```python
from build123d import *

# Parameters (mm, degrees)
SKETCH_1_R          = 210
SKETCH_1_R_2        = 203
EXTRUDE_2_DEPTH     = 174
EXTRUDE_START       = -174
EXTRUDE_4_DEPTH     = 174
CUT_EXTRUDE_1_DEPTH = 654
EXTRUDE_5_DEPTH     = 174
EXTRUDE_6_DEPTH     = 174
EXTRUDE_7_DEPTH     = 174
EXTRUDE_8_DEPTH     = 174
EXTRUDE_9_DEPTH     = 174
SKETCH_11_R         = 55
CUT_EXTRUDE_4_DEPTH = 221.5
CUT_EXTRUDE_5_DEPTH = 87


with BuildPart() as part:
    # 草图1 → 凸台-拉伸2 (new body)
    with BuildSketch(Plane.XY):
        Circle(SKETCH_1_R)
        Circle(SKETCH_1_R_2, mode=Mode.SUBTRACT)
    extrude(amount=EXTRUDE_2_DEPTH)

    # 草图2 → 凸台-拉伸4 (add)
    with BuildSketch(Plane.XY.offset(174).offset(EXTRUDE_START)):
        with BuildLine():
            Line((-170.735431044, -102), (-173.735431044, -102))
            Line((-173.735431044, -102), (-175.513532242, -102))
            ThreePointArc((-175.513532242, -102), (-174.63092392, -103.50381834), (-173.735431044, -105))
            Line((-173.735431044, -105), (-170.735431044, -105))
            Line((-170.735431044, -105), (-170.735431044, -102))
        make_face()
        with BuildLine():
            ThreePointArc((173.735431044, -105), (174.63092392, -103.50381834), (175.513532242, -102))
            Line((175.513532242, -102), (173.735431044, -102))
            Line((173.735431044, -102), (170.735431044, -102))
            Line((170.735431044, -102), (170.735431044, -105))
            Line((170.735431044, -105), (173.735431044, -105))
        make_face()
    extrude(amount=EXTRUDE_4_DEPTH)

    # 草图3 → 切除-拉伸1 (cut)
    with BuildSketch(Plane.XY.offset(174)):
        Polygon((-170.735431044, -102), (238.333646515, -102), (254.334169784, 272.292523591), (-334.569415043, 221.85110305), (-306.830562533, -102), align=None)
    extrude(amount=-CUT_EXTRUDE_1_DEPTH, mode=Mode.SUBTRACT)

    # 草图5 → 凸台-拉伸5 (add)
    with BuildSketch(Plane.XY.offset(174).offset(EXTRUDE_START)):
        with BuildLine():
            Line((-120, -209.75), (-10.243900624, -209.75))
            ThreePointArc((-10.243900624, -209.75), (-67.755470707, -198.769203322), (-120, -172.336879396))
            Line((-120, -172.336879396), (-120, -209.75))
        make_face()
        with BuildLine():
            ThreePointArc((120, -172.336879396), (67.755470707, -198.769203322), (10.243900624, -209.75))
            Line((10.243900624, -209.75), (120, -209.75))
            Line((120, -209.75), (120, -172.336879396))
        make_face()
    extrude(amount=EXTRUDE_5_DEPTH)

    # 草图6 → 凸台-拉伸6 (add)
    with BuildSketch(Plane.XY.offset(174).offset(EXTRUDE_START)):
        with BuildLine():
            Line((-175.513532242, -102), (-166.195667814, -102))
            ThreePointArc((-166.195667814, -102), (0, -195), (166.195667814, -102))
            Line((166.195667814, -102), (175.513532242, -102))
            ThreePointArc((175.513532242, -102), (0, -203), (-175.513532242, -102))
        make_face()
    extrude(amount=EXTRUDE_6_DEPTH)

    # 草图7 → 凸台-拉伸7 (add)
    with BuildSketch(Plane.XY.offset(174).offset(EXTRUDE_START)):
        with BuildLine():
            Line((-166.933126535, -92), (-166.933126535, -95))
            Line((-166.933126535, -95), (-170.293863659, -95))
            ThreePointArc((-170.293863659, -95), (0, -195), (170.293863659, -95))
            Line((170.293863659, -95), (166.933126535, -95))
            Line((166.933126535, -95), (166.933126535, -92))
            Line((166.933126535, -92), (171.933126535, -92))
            Line((171.933126535, -92), (188.496850106, -92))
            ThreePointArc((188.496850106, -92), (0, -209.75), (-188.496850106, -92))
            Line((-188.496850106, -92), (-171.933126535, -92))
            Line((-171.933126535, -92), (-166.933126535, -92))
        make_face()
    extrude(amount=EXTRUDE_7_DEPTH)

    # 草图8 → 凸台-拉伸8 (add)
    with BuildSketch(Plane(origin=(0, 0, 0), x_dir=(-1, 0, 0), z_dir=(0, 0, -1))):
        with BuildLine():
            Line((166.933126535, -92), (163.933126535, -92))
            Line((163.933126535, -92), (163.933126535, -99))
            Line((163.933126535, -99), (168, -99))
            ThreePointArc((168, -99), (169.158755456, -97.006780447), (170.293863659, -95))
            Line((170.293863659, -95), (166.933126535, -95))
            Line((166.933126535, -95), (166.933126535, -92))
        make_face()
        with BuildLine():
            Line((-166.933126535, -95), (-170.293863659, -95))
            ThreePointArc((-170.293863659, -95), (-169.158755456, -97.006780447), (-168, -99))
            Line((-168, -99), (-163.933126535, -99))
            Line((-163.933126535, -99), (-163.933126535, -92))
            Line((-163.933126535, -92), (-166.933126535, -92))
            Line((-166.933126535, -92), (-166.933126535, -95))
        make_face()
    extrude(amount=-EXTRUDE_8_DEPTH)

    # 草图9 → 凸台-拉伸9 (add)
    with BuildSketch(Plane.XY.offset(174).offset(EXTRUDE_START)):
        with BuildLine():
            ThreePointArc((10.243900624, -209.75), (5.123475383, -209.937490697), (0, -210))
            Line((0, -210), (0, -225))
            Line((0, -225), (18.007375678, -225))
            Line((18.007375678, -225), (120, -225))
            Line((120, -225), (120, -209.75))
            Line((120, -209.75), (10.243900624, -209.75))
        make_face()
        with BuildLine():
            Line((0, -225), (0, -210))
            ThreePointArc((0, -210), (-5.123475383, -209.937490697), (-10.243900624, -209.75))
            Line((-10.243900624, -209.75), (-120, -209.75))
            Line((-120, -209.75), (-120, -225))
            Line((-120, -225), (0, -225))
        make_face()
    extrude(amount=EXTRUDE_9_DEPTH)

    # 草图11 → 切除-拉伸4 (cut)
    with BuildSketch(Plane(origin=(0, 0, 0), x_dir=(1, 0, 0), z_dir=(0, 1, 0))):
        with Locations(Location((0, -87, 0), (0, 0, 270))):
            Circle(SKETCH_11_R)
    extrude(amount=-CUT_EXTRUDE_4_DEPTH, mode=Mode.SUBTRACT)

    # 草图10 → 切除-拉伸5 (cut)
    with BuildSketch(Plane.XY.offset(174)):
        Polygon((5, -221.5), (-5, -221.5), (-5, -211.5), (0, -211.5), (5, -211.5), align=None)
    extrude(amount=-CUT_EXTRUDE_5_DEPTH, mode=Mode.SUBTRACT)


solid = part.part
```
Geometry check sheet. Reference: the model listing, model coordinates, mm. A direction names the side the tool comes from. Coordinates: 2 decimals unless noted, no trailing zeros. Order: outer loops, then holes, each group sorted by start corner. A loop starts at its lowest first (then second) coordinate and runs counter-clockwise, first axis right, second up. Notation, with made-up numbers: (71, 39) - (118, 39) arc R27 ccw to (118, 69) - close; hole circle Ø8 at (54.5, -13). An arc over 180 degrees is marked (long way). Answer as a JSON object with one key per item and string values. Group by question number.
Item 1: Sectioned sample at D-D, the plane z = 87. Record the cut outline in (x, y).
Item 2: Scan lines: probe 1 along Z at (x, y) = (0, -202); probe 2 along X at (y, z) = (-207.5, 87); probe 3 along X at (y, z) = (-210.5, 14). Record each from-to range of solid material in increasing order.
Item 3: Depth check by flat-ended pin: pin 1 Ø5 at (y, z) = (-218, 150.5) entering from -X; pin 2 Ø5 at (y, z) = (-191, 55) entering from +X; pin 3 Ø4 at (y, z) = (-111, 88.5) entering from -X. Enter the tip coordinate at first touch or a pass-through.
Item 4: Sectioned sample at C-C, the plane y = -153. Record the cut outline in (x, z), and give its area (3 significant figures).
Item 5: Sectioned sample at B-B, the plane z = 156.5. Record the cut outline in (x, y).
Item 6: Sectioned sample at A-A, the plane x = 0. Record the cut outline in (y, z), and give its area (4 significant figures).
Item 7: Tool access check on faces 1 (the face through (120, -199, 86)), 2 (the face through (5, -216, 158)), 3 (the face through (-163.933, -95, 86)), 4 (the face through (-120, -198, 86)). Record the directions out of +Z, -Z, +X, -X, +Y, -Y that give a thin tool (end or side, any length) a straight path to the whole face; none if there is none.
Item 8: Draft check along X on faces 5 (the face through (-176, -92, 86)), 6 (the face through (155.35, -141.3, 85.78)), 7 (the face through (2.418, -207.872, 32.053)). Enter one of: +X half, -X half, draft (parallel to the pull), parting line (faces both ways), or undercut.
Resolved:
{
 "1": {"outline": "(-188.5, -92) arc R209.75 ccw to (-183.28, -102) - (-183.56, -102) arc R210 ccw to (-120, -172.34) - (-120, -225) - (120, -225) - (120, -172.34) arc R210 ccw to (183.56, -102) - (183.28, -102) arc R209.75 ccw to (188.5, -92) - (163.93, -92) - (163.93, -99) - (168, -99) arc R195 cw to (55, -187.08) - (55, -221.5) - (-55, -221.5) - (-55, -187.08) arc R195 cw to (-168, -99) - (-163.93, -99) - (-163.93, -92) - close"},
 "2": {"probe 1": "0 to 32, 142 to 174", "probe 2": "-120 to -55, 55 to 120", "probe 3": "-120 to 120"},
 "3": {"pin 1": "x = -120", "pin 2": "x = 120", "pin 3": "x = -179.5"},
 "4": {"outline": "(-143.84, 0) - (-120.9, 0) - (-120.9, 174) - (-143.84, 174) - close; (120.9, 0) - (143.84, 0) - (143.84, 174) - (120.9, 174) - close", "area": "7,990 mm^2"},
 "5": {"outline": "(-188.5, -92) arc R209.75 ccw to (-183.28, -102) - (-183.56, -102) arc R210 ccw to (-120, -172.34) - (-120, -225) - (120, -225) - (120, -172.34) arc R210 ccw to (183.56, -102) - (183.28, -102) arc R209.75 ccw to (188.5, -92) - (163.93, -92) - (163.93, -99) - (168, -99) arc R195 cw to (-168, -99) - (-163.93, -99) - (-163.93, -92) - close; hole (-5, -221.5) - (5, -221.5) - (5, -211.5) - (-5, -211.5) - close"},
 "6": {"outline": "(-225, 0) - (-195, 0) - (-195, 32) - (-221.5, 32) - (-221.5, 174) - (-225, 174) - close; (-211.5, 142) - (-195, 142) - (-195, 174) - (-211.5, 174) - close", "area": "1,985 mm^2"},
 "7": {"face 1": "+Z, -Z, +X, -Y", "face 2": "+Z", "face 3": "+Z, -Z, +Y", "face 4": "+Z, -Z, -X, -Y"},
 "8": {"face 5": "draft", "face 6": "+X half", "face 7": "undercut"}
}
